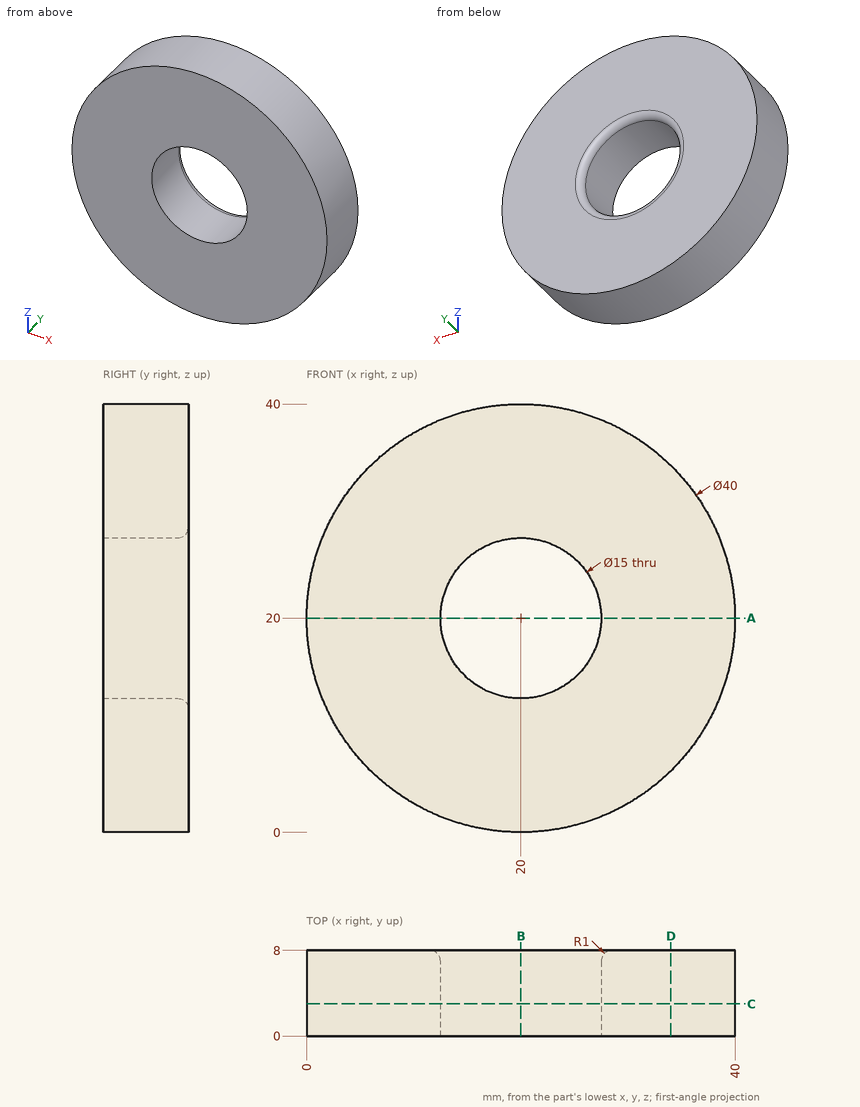
The figure shows three views and two pictorial views of one solid part (mm, origin at its lowest corner). Answer the questions. Give positions to 0.01 mm unless a question says otherwise; leave off trailing zeros. Order: outer loops, then holes, each group sorted by start corner. A loop starts at its lowest first (then second) coordinate and runs counter-clockwise, first axis right, second up. Notation, with made-up numbers: (71, 73) -> (111, 73) arc R20 cw to (111, 108) -> close; hole circle Ø11 at (83, 49.5). An arc over 180 degrees is marked (long way). Answer as CSV lines item,"result". Start each with the question number.
Q1. Given pin 1 (3 mm diameter, centred on y = 3.5, z = 30.5, fed in from -X); pin 2 (2 mm diameter, centred on x = 9.5, y = 2, fed in from -Z); pin 3 (1.5 mm diameter, centred on y = 6.5, z = 34, fed in from +X), each flat-ended and moving along its own axis, determine where each tip first touches the part or whether it passes through.
Q2. A cutting plane is placed at B-B (x = 20). Determine the outline of the cut face in (y, z).
Q3. A cutting plane is placed at D-D (x = 34). Determine the outline of the cut face in (y, z), then the cut area to 3 significant figures.
Q4. Find the intervals of material crossed by L1, parallel to Z at x = 20, y = 3.5; L2, parallel to Z at x = 16.5, y = 3.25, in increasing order.
Q5. A cutting plane is placed at C-C (y = 3). Determine the outline of the cut face in (x, z).
Q6. A cutting plane is placed at A-A (z = 20). Determine the outline of the cut face in (x, y), then the cut area to 3 significant figures.
Results found:
1,pin 1,"x = 2.14"
1,pin 2,"z = 2.4"
1,pin 3,"x = 34.98"
2,outline,"(0, 0) -> (8, 0) -> (8, 11.5) arc R1 ccw to (7, 12.5) -> (0, 12.5) -> close; (0, 27.5) -> (7, 27.5) arc R1 ccw to (8, 28.5) -> (8, 40) -> (0, 40) -> close"
3,outline,"(0, 5.72) -> (8, 5.72) -> (8, 34.28) -> (0, 34.28) -> close"
3,area,"229 mm2"
4,L1,"0 to 12.5, 27.5 to 40"
4,L2,"0.31 to 13.37, 26.63 to 39.69"
5,outline,"circle Ø40 at (20, 20); hole circle Ø15 at (20, 20)"
6,outline,"(0, 0) -> (12.5, 0) -> (12.5, 7) arc R1 ccw to (11.5, 8) -> (0, 8) -> close; (27.5, 0) -> (40, 0) -> (40, 8) -> (28.5, 8) arc R1 ccw to (27.5, 7) -> close"
6,area,"200 mm2"
